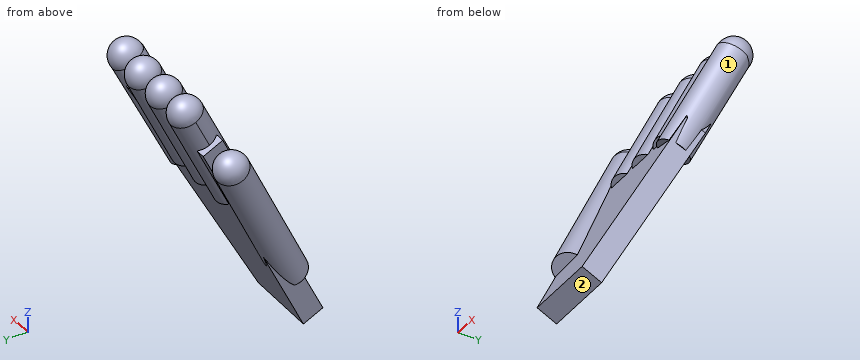
```python
from build123d import *

# Parameters (mm, degrees)
CYLINDER076_R                     = 1.5
CYLINDER076_DEPTH                 = 10
CYLINDER076_ROLL_ANGLE            = -86.804178
CYLINDER076_PITCH_ANGLE           = 18.403125
CYLINDER076_PLACEMENT_ANGLE       = 19.43972
CYLINDER074_R                     = 1.5
CYLINDER074_DEPTH                 = 10
CYLINDER075_R                     = 1.5
CYLINDER075_DEPTH                 = 10
CYLINDER078_R                     = 1.5
CYLINDER078_DEPTH                 = 10
CYLINDER077_R                     = 1.5
CYLINDER077_DEPTH                 = 17
CYLINDER077_ROLL_ANGLE            = 87.960425
CYLINDER077_PITCH_ANGLE           = -11.302952
CYLINDER077_PLACEMENT_ANGLE       = -10.91002
BOX026_W                          = 10
BOX026_H                          = 19
BOX026_DEPTH                      = 10
BOX026_PLACEMENT_ANGLE            = 16
BOX025_W                          = 11
BOX025_H                          = 22
BOX025_DEPTH                      = 2
PART_MIRRORING003_PLACEMENT_ANGLE = 65


with BuildPart() as cylindre072:
    # Cylinder076 → Cylinder076 (new body)
    with BuildSketch(Plane.XY):
        Circle(CYLINDER076_R)
    extrude(amount=CYLINDER076_DEPTH)


with BuildPart() as cylindre072_1:
    # Cylinder076 roll: moved
    add(cylindre072.part.rotate(Axis((0, 0, 0), (1, 0, 0)), CYLINDER076_ROLL_ANGLE))


with BuildPart() as cylindre072_2:
    # Cylinder076 pitch: moved
    add(cylindre072_1.part.rotate(Axis((0, 0, 0), (0, 1, 0)), CYLINDER076_PITCH_ANGLE))


with BuildPart() as cylindre072_3:
    # Cylinder076 placement: moved
    add(cylindre072_2.part.moved(Location((-5, 26, -135))).rotate(Axis((-5, 26, -135), (0, 0, 1)), CYLINDER076_PLACEMENT_ANGLE))


with BuildPart() as obj1:
    # Sphere004 → Sphere004 (revolve)
    with BuildSketch(Plane(origin=(-8.15, 35.5, -134.5), x_dir=(1, 0, 0), z_dir=(0, -1, 0))):
        with BuildLine():
            ThreePointArc((0, -1.5), (1.5, 0), (0, 1.5))
            Line((0, 1.5), (0, -1.5))
        make_face()
    revolve(axis=Axis((-8.15, 35.5, -134.5), (0, 0, 1)))


with BuildPart() as cylindre070:
    # Cylinder074 → Cylinder074 (new body)
    with BuildSketch(Plane(origin=(-4, 37, -135), x_dir=(1, 0, 0), z_dir=(0, -1, 0))):
        Circle(CYLINDER074_R)
    extrude(amount=CYLINDER074_DEPTH)


with BuildPart() as obj2:
    # Sphere003 → Sphere003 (revolve)
    with BuildSketch(Plane(origin=(-4, 37, -135), x_dir=(1, 0, 0), z_dir=(0, -1, 0))):
        with BuildLine():
            ThreePointArc((0, -1.5), (1.5, 0), (0, 1.5))
            Line((0, 1.5), (0, -1.5))
        make_face()
    revolve(axis=Axis((-4, 37, -135), (0, 0, 1)))


with BuildPart() as cylindre071:
    # Cylinder075 → Cylinder075 (new body)
    with BuildSketch(Plane(origin=(-1, 37, -135), x_dir=(1, 0, 0), z_dir=(0, -1, 0))):
        Circle(CYLINDER075_R)
    extrude(amount=CYLINDER075_DEPTH)


with BuildPart() as obj3:
    # Sphere002 → Sphere002 (revolve)
    with BuildSketch(Plane(origin=(-1, 37, -135), x_dir=(1, 0, 0), z_dir=(0, -1, 0))):
        with BuildLine():
            ThreePointArc((0, -1.5), (1.5, 0), (0, 1.5))
            Line((0, 1.5), (0, -1.5))
        make_face()
    revolve(axis=Axis((-1, 37, -135), (0, 0, 1)))


with BuildPart() as cylindre074:
    # Cylinder078 → Cylinder078 (new body)
    with BuildSketch(Plane(origin=(2, 37, -135), x_dir=(1, 0, 0), z_dir=(0, -1, 0))):
        Circle(CYLINDER078_R)
    extrude(amount=CYLINDER078_DEPTH)


with BuildPart() as obj4:
    # Sphere001 → Sphere001 (revolve)
    with BuildSketch(Plane(origin=(2, 37, -135), x_dir=(1, 0, 0), z_dir=(0, -1, 0))):
        with BuildLine():
            ThreePointArc((0, -1.5), (1.5, 0), (0, 1.5))
            Line((0, 1.5), (0, -1.5))
        make_face()
    revolve(axis=Axis((2, 37, -135), (0, 0, 1)))


with BuildPart() as cylindre073:
    # Cylinder077 → Cylinder077 (new body)
    with BuildSketch(Plane.XY):
        Circle(CYLINDER077_R)
    extrude(amount=CYLINDER077_DEPTH)


with BuildPart() as cylindre073_1:
    # Cylinder077 roll: moved
    add(cylindre073.part.rotate(Axis((0, 0, 0), (1, 0, 0)), CYLINDER077_ROLL_ANGLE))


with BuildPart() as cylindre073_2:
    # Cylinder077 pitch: moved
    add(cylindre073_1.part.rotate(Axis((0, 0, 0), (0, 1, 0)), CYLINDER077_PITCH_ANGLE))


with BuildPart() as cylindre073_3:
    # Cylinder077 placement: moved
    add(cylindre073_2.part.moved(Location((6, 33, -135))).rotate(Axis((6, 33, -135), (0, 0, 1)), CYLINDER077_PLACEMENT_ANGLE))


with BuildPart() as obj5:
    # Sphere005 → Sphere005 (revolve)
    with BuildSketch(Plane(origin=(6, 33, -135), x_dir=(1, 0, 0), z_dir=(0, -1, 0))):
        with BuildLine():
            ThreePointArc((0, -1.5), (1.5, 0), (0, 1.5))
            Line((0, 1.5), (0, -1.5))
        make_face()
    revolve(axis=Axis((6, 33, -135), (0, 0, 1)))


with BuildPart() as cube026:
    # Box026 → Box026 (new body)
    with BuildSketch(Plane.XY):
        with Locations((5, 9.5)):
            Rectangle(BOX026_W, BOX026_H)
    extrude(amount=BOX026_DEPTH)


with BuildPart() as cube026_1:
    # Box026 placement: moved
    add(cube026.part.moved(Location((-12, 9, -144))).rotate(Axis((-12, 9, -144), (0, 0, 1)), BOX026_PLACEMENT_ANGLE))


with BuildPart() as fusion040:
    # Box025 → Box025 (new body)
    with BuildSketch(Plane(origin=(-7, 12, -136), x_dir=(1, 0, 0), z_dir=(0, 0, 1))):
        with Locations((5.5, 11)):
            Rectangle(BOX025_W, BOX025_H)
    extrude(amount=BOX025_DEPTH)

    # Cut042: cut Cube026
    add(cube026_1.part, mode=Mode.SUBTRACT)

    # Fusion040: union Cylindre072, obj1, Cylindre070, obj2, Cylindre071, obj3, Cylindre074, obj4, Cylindre073, obj5
    add(cylindre072_3.part)
    add(obj1.part)
    add(cylindre070.part)
    add(obj2.part)
    add(cylindre071.part)
    add(obj3.part)
    add(cylindre074.part)
    add(obj4.part)
    add(cylindre073_3.part)
    add(obj5.part)


with BuildPart() as part_mirroring003:
    # Part__Mirroring003: instance of Fusion040
    add(fusion040.part.mirror(Plane(origin=(0, 0, 0), x_dir=(0, -1, 0), z_dir=(1, 0, 0))))


with BuildPart() as part_mirroring003_1:
    # Part__Mirroring003 placement: moved
    add(part_mirroring003.part.moved(Location((17, -107, -42))).rotate(Axis((17, -107, -42), (1, 0, 0)), PART_MIRRORING003_PLACEMENT_ANGLE))


solid = part_mirroring003_1.part
```
Build history of the part. All positions in model axes, mm. Face numbers are marked on the shaded views. Round coordinates to 2 decimals unless told otherwise and drop trailing zeros. Loops run counter-clockwise (first coordinate to the right, second up) from the corner with the lowest first, then second, coordinate; pieces in that order, holes last.
Item 1: Two-plate mould, pull along X, no slides. Class the marked faces 1 and 2: released by +X, released by -X, zero draft, split by the parting line, or undercut.
Item 2: Saw through at A-A (x = 17.5). List the corners of the cut face in (y, z), then the cut area to 3 significant figures.
Item 3: Saw through at B-B (x = 20.25). List the corners of the cut face in (y, z).
Item 4: Drill centre lines: line 1 along X through (y, z) = (29.5, -70); line 2 along Z through (x, y) = (13.5, 25.75); line 3 along Y through (x, z) = (16.5, -78). Where is each one in solid material? Low to high.
Item 5: Pin check, flat tips, straight feed: P1, Ø0.7, axis at y = 28, z = -74, coming from the +X side; P2, Ø1.1, axis at y = 28.5, z = -71.5, coming from the -X side; P3, Ø2, axis at x = 17, y = 28, coming from the -Z side; P4, Ø6, axis at x = 18.5, y = 28, coming from the +Z side. Stop position of each tip, or through.
Worked answers:
1. face 1: undercut
1. face 2: zero draft
2. outline: (19.52, -87.76) - (21.33, -88.6) - (27.67, -75.01) - (28.04, -75.18) - (32.27, -66.12) arc R1.41 ccw to (29.71, -64.92) - (25.48, -73.99) - (25.86, -74.16) - close
2. area: 61.4 mm2
3. outline: (20.69, -85.25) - (22.5, -86.09) - (27.67, -75.01) - (27.94, -75.13) - (32.17, -66.07) arc R1.3 ccw to (29.81, -64.97) - (25.58, -74.03) - (25.86, -74.16) - close
4. line 1: x = 9.72 to 12.55, 13 to 25.35
4. line 2: z = -79.3 to -74.25
4. line 3: y = 24.07 to 26.27
5. P1: stops at x = 24.13
5. P2: stops at x = 9.87
5. P3: stops at z = -76.44
5. P4: stops at z = -64.02
